Answer from the drawing. Dimensions are ordinates in mm from the lowest x, y and z of the part. A direction names the side the tool comes from. Round coordinates to 2 decimals unless told otherwise and drop trailing zeros. Write each loop counter-clockwise with the first axis right and the second up, starting at its lowest first coordinate (ties: lowest second). Pieces come first, ordered by that corner, then holes. Notation, with made-up numbers: (42, 27) - (81, 27) arc R19 ccw to (81, 58) - close; hole circle Ø1 at (58.25, -33). An arc over 180 degrees is marked (long way). Use a Markdown table: item, result. Add a question column.
1) Each of these flat-tipped pins is pushed along its axis until it touches: P1, Ø0.8, axis at y = 2, z = 47.5, coming from the +X side; P2, Ø3, axis at x = 15, z = 1, coming from the +Y side; P3, Ø3, axis at x = 11, y = 2, coming from the +Z side; P4, Ø12, axis at y = 33, z = 39.5, coming from the +X side. Where does it stop, or does it pass through?
2) A tool of negligible diameter and unlimited length cuts with its end or side. For the marked faces 1, 2 and 3, from which of +Z, -Z, +X, -X, +Y, -Y can it reach the whole face along a straight path? Write none if from no direction.
3) Determine the mould class of the marked faces 4, 5 and 6 for opening direction Y: +Y half, -Y half, draft (parallel to the pull), parting line (faces both ways), or undercut.
4) A cutting plane is placed at D-D (y = 18). Give the vertices of the cut face in (x, z).
5) A cutting plane is placed at C-C (x = 10.5). Give the vertices of the cut face in (y, z).
6) Find the intervals of material crossed by probe 1 along X at (y, z) = (25, 1); probe 2 along Z at (x, y) = (10.5, 34); probe 3 along Y at (x, z) = (16.5, 33.5), in increasing order. Write a range as from..to.
7) A cutting plane is placed at A-A (z = 47). Give the vertices of the cut face in (x, y) (1 decimal).
8) A cutting plane is placed at B-B (z = 36). Give the vertices of the cut face in (x, y), then the cut area to 3 significant figures.
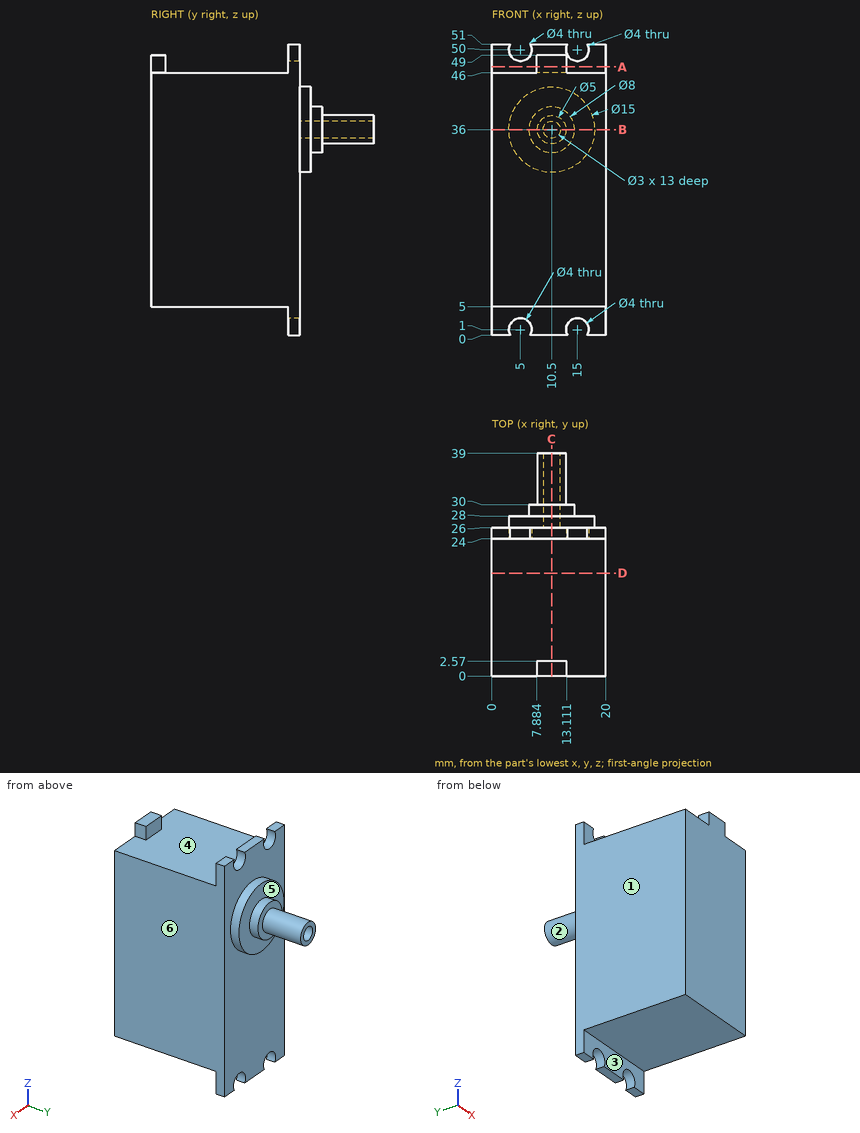
Entries:
| question | item | result |
|---|---|---|
| 1 | P1 | stops at x = 13.11 |
| 1 | P2 | passes through |
| 1 | P3 | stops at z = 49 |
| 1 | P4 | stops at x = 18 |
| 2 | face 1 | +Z, -Z, -X, +Y, -Y |
| 2 | face 2 | +Y |
| 2 | face 3 | -Z, +X, -X, -Y |
| 3 | face 4 | undercut |
| 3 | face 5 | +Y half |
| 3 | face 6 | draft |
| 4 | outline | (0, 5) - (20, 5) - (20, 46) - (0, 46) - close |
| 5 | outline | (0, 5) - (24, 5) - (24, 0) - (26, 0) - (26, 28.5) - (28, 28.5) - (28, 32) - (30, 32) - (30, 33.5) - (39, 33.5) - (39, 34.5) - (26, 34.5) - (26, 37.5) - (39, 37.5) - (39, 38.5) - (30, 38.5) - (30, 40) - (28, 40) - (28, 43.5) - (26, 43.5) - (26, 51) - (24, 51) - (24, 46) - (2.57, 46) - (2.57, 49) - (0, 49) - close |
| 6 | probe 1 | x = 0..3, 7..13, 17..20 |
| 6 | probe 2 | z = 33.5..34.5, 37.5..38.5 |
| 6 | probe 3 | y = 0..28 |
| 7 | outline | (0, 24) - (20, 24) - (20, 26) - (0, 26) - close; (7.9, 0) - (13.1, 0) - (13.1, 2.6) - (7.9, 2.6) - close |
| 8 | outline | (0, 0) - (20, 0) - (20, 26) - (18, 26) - (18, 28) - (14.5, 28) - (14.5, 30) - (13, 30) - (13, 39) - (12, 39) - (12, 26) - (9, 26) - (9, 39) - (8, 39) - (8, 30) - (6.5, 30) - (6.5, 28) - (3, 28) - (3, 26) - (0, 26) - close |
| 8 | area | 572 mm² |
